from build123d import *

# Parameters (mm, degrees)
F0_R     = 2.75
F1_DEPTH = 5
F2_R     = 3.05
F3_DEPTH = 0.5
F4_R     = 2
F5_DEPTH = 25
F6_W     = 2
F6_H     = 8.049181
F7_DEPTH = 4.5
F8_W     = 2
F8_H     = 8.049182
F9_DEPTH = 4.5


with BuildPart() as f1:
    # F0 (on Top) → F1 (new body, symmetric)
    with BuildSketch(Plane.XY):
        Circle(F0_R)
    extrude(amount=F1_DEPTH, both=True)

    # F2 (on Top) → F3 (join, symmetric)
    with BuildSketch(Plane.XY):
        Circle(F2_R)
    extrude(amount=F3_DEPTH, both=True)

    # F4 (on face) → F5 (cut)
    with BuildSketch(Plane.XY.offset(5)):
        Circle(F4_R)
    extrude(amount=-F5_DEPTH, mode=Mode.SUBTRACT)

    # F6 (on face) → F7 (cut)
    with BuildSketch(Plane.XY.offset(5)):
        with Locations((0, -0.130544)):
            Rectangle(F6_W, F6_H)
    extrude(amount=-F7_DEPTH, mode=Mode.SUBTRACT)

    # F8 (on face) → F9 (cut)
    with BuildSketch(Plane(origin=(0, 0, -5), x_dir=(1, 0, 0), z_dir=(0, 0, -1))):
        Rectangle(F8_W, F8_H)
    extrude(amount=-F9_DEPTH, mode=Mode.SUBTRACT)


solid = f1.part
Could you check a few things on this model? Use its own coordinates, in mm. A direction names the side the tool comes from. Give positions to 0.01 mm unless a question says otherwise; leave off trailing zeros. Order: outer loops, then holes, each group sorted by start corner. A loop starts at its lowest first (then second) coordinate and runs counter-clockwise, first axis right, second up. Notation, with made-up numbers: (16.25, 64) - (25.25, 64) arc R27 ccw to (25.25, 95) - close; hole circle Ø10 at (38, -2). An arc over 180 degrees is marked (long way). Return JSON: item names as keys, results as strings. Group by question number.
Q1. Which directions (+Z, -Z, +X, -X, +Y, -Y) give clear straight access to the entire face, cutting with the end or side of a thin tool? Please do faces 1 (the face through (1, -2, 3)), 2 (the face through (-1, -2, -3)), 3 (the face through (2.75, -0.05, 2.78)).
Q2. Suppose I cut it at A-A, the plane z = -3.5. Please give me the cut outline in (x, y).
Q3. Suppose I cut it at B-B, the plane x = 0. Please give me the cut outline in (y, z), and give its area (3 significant figures).
Q4. Please list where these lines run through material, in increasing order: line 1 along Y through (x, z) = (0, 0); line 2 along X through (y, z) = (0, 1); line 3 along X through (y, z) = (-0.5, 0). Write a range as [from, to].
Q5. Thinking about a two-plate mould opening in X: for faces 4 (the face through (1, -2, -3)), 5 (the face through (-2.75, 0.05, -2.72)), 6 (the face through (2.75, -0.05, -2.72)), which applies, pulls with the +X half, pulls with the -X half, needs draft (parallel to the pull), parting line crosses it, or undercut?
Q6. Suppose I cut it at C-C, the plane y = 0. Please give me the cut outline in (x, z).
Q7. Will these pins go through, and if not, where does the flat tip stop? pin 1 Ø0.7 at (y, z) = (-2, -3.5) entering from -X; pin 2 Ø0.9 at (y, z) = (2, 2.5) entering from -X; pin 3 Ø2 at (y, z) = (-1.5, -0.5) entering from -X.
Q8. Suppose I cut it at D-D, the plane x = 2.25. Please give me the cut outline in (y, z).
Resolved:
{
 "1": {"face 1": "+Z, +Y, -Y", "face 2": "-Z, +Y, -Y", "face 3": "+Z, +X"},
 "2": {"outline": "(-1, -2.56) - (-1, -1.73) arc R2 cw to (-1, 1.73) - (-1, 2.56) arc R2.75 ccw to start; (1, -2.56) arc R2.75 ccw to (1, 2.56) - (1, 1.73) arc R2 cw to (1, -1.73) - close"},
 "3": {"outline": "(-3.05, -0.5) - (-2, -0.5) - (-2, 0.5) - (-3.05, 0.5) - close; (2, -0.5) - (3.05, -0.5) - (3.05, 0.5) - (2, 0.5) - close", "area": "2.10 mm2"},
 "4": {"line 1": "y = [-3.05, -2], [2, 3.05]", "line 2": "x = [-2.75, -2], [2, 2.75]", "line 3": "x = [-3.01, -1.94], [1.94, 3.01]"},
 "5": {"face 4": "undercut", "face 5": "pulls with the -X half", "face 6": "pulls with the +X half"},
 "6": {"outline": "(-3.05, -0.5) - (-2.75, -0.5) - (-2.75, -5) - (-2, -5) - (-2, 5) - (-2.75, 5) - (-2.75, 0.5) - (-3.05, 0.5) - close; (2, -5) - (2.75, -5) - (2.75, -0.5) - (3.05, -0.5) - (3.05, 0.5) - (2.75, 0.5) - (2.75, 5) - (2, 5) - close"},
 "7": {"pin 1": "stops at x = -2.2", "pin 2": "stops at x = -2.27", "pin 3": "stops at x = -3.01"},
 "8": {"outline": "(-2.06, -0.5) - (-1.58, -0.5) - (-1.58, -5) - (1.58, -5) - (1.58, -0.5) - (2.06, -0.5) - (2.06, 0.5) - (1.58, 0.5) - (1.58, 5) - (-1.58, 5) - (-1.58, 0.5) - (-2.06, 0.5) - close"}
}
